Source: CAD feature listing. Evaluate the final solid. Frame: model axes, mm. Face numbers are marked on the shaded views. A direction names the side the tool comes from. Give positions to 0.01 mm unless a question says otherwise; leave off trailing zeros. Loops run counter-clockwise (first coordinate to the right, second up) from the corner with the lowest first, then second, coordinate; pieces in that order, holes last.
from build123d import *

# Parameters (mm, degrees)
IZIM1_R                     = 25
IZIM1_R_2                   = 7.5
Y_KSEKLIK_EKSTR_ZYON1_DEPTH = 80.5
IZIM2_R                     = 16
KES_EKSTR_ZYON1_DEPTH       = 9


with BuildPart() as part:
    # Çizim1 → Yükseklik-Ekstrüzyon1 (new, symmetric)
    with BuildSketch(Plane(origin=(0, 0, 0), x_dir=(0, 0, -1), z_dir=(1, 0, 0))):
        Circle(IZIM1_R)
        Circle(IZIM1_R_2, mode=Mode.SUBTRACT)
    extrude(amount=Y_KSEKLIK_EKSTR_ZYON1_DEPTH, both=True)

    # Çizim2 → Kes-Ekstrüzyon1 (cut)
    with BuildSketch(Plane(origin=(80.5, 0, 0), x_dir=(0, 0, -1), z_dir=(1, 0, 0))):
        Circle(IZIM2_R)
    kes_ekstr_zyon1 = extrude(amount=-KES_EKSTR_ZYON1_DEPTH, mode=Mode.SUBTRACT)

    # Aynalama1: Kes-Ekstrüzyon1 across plane
    add(kes_ekstr_zyon1.mirror(Plane(origin=(0, 0, 0), x_dir=(0, 0, 1), z_dir=(1, 0, 0))), mode=Mode.SUBTRACT)


solid = part.part
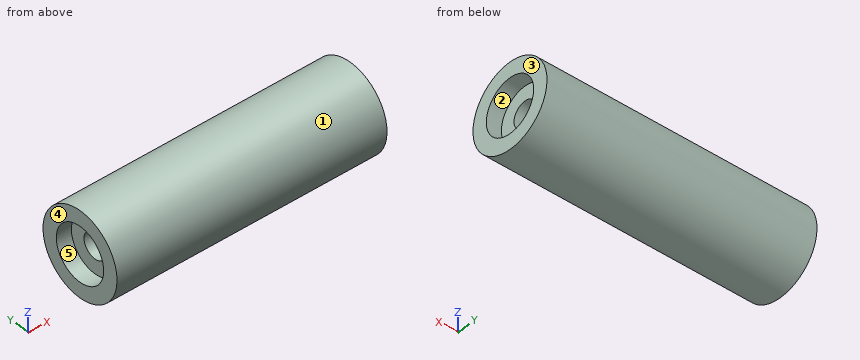
1) Pull-direction query (Z, two-part tool) for the marked faces 1, 2 and 3; classes: released by +Z, released by -Z, zero draft, split by the parting line, or undercut.
Checks:
face 1: split by the parting line
face 2: undercut
face 3: zero draft
2) Reachability of the marked faces 4 and 5 from +Z, -Z, +X, -X, +Y, -Y: full face, straight path, thin tool, end or side. Return the list, or none.
Checks:
face 4: +Z, -Z, -X, +Y, -Y
face 5: -X
3) Ray query, probe 1 along Y at (x, z) = (11.5, 0); probe 2 along Y at (x, z) = (-73, 0); probe 3 along X at (y, z) = (0.5, -13.5). Return the intervals inside material, ascending.
Checks:
probe 1: y = -25 to -7.5, 7.5 to 25
probe 2: y = -25 to -16, 16 to 25
probe 3: x = -71.5 to 71.5
4) Cut plane A-A (z = 0). Return loops of the section in (x, y).
Checks:
outline: (-80.5, -25) - (80.5, -25) - (80.5, -16) - (71.5, -16) - (71.5, -7.5) - (-71.5, -7.5) - (-71.5, -16) - (-80.5, -16) - close; (-80.5, 16) - (-71.5, 16) - (-71.5, 7.5) - (71.5, 7.5) - (71.5, 16) - (80.5, 16) - (80.5, 25) - (-80.5, 25) - close
5) Cut plane D-D (y = -14). Return loops of the section in (x, z).
Checks:
outline: (-80.5, -20.71) - (80.5, -20.71) - (80.5, -7.75) - (71.5, -7.75) - (71.5, 7.75) - (80.5, 7.75) - (80.5, 20.71) - (-80.5, 20.71) - (-80.5, 7.75) - (-71.5, 7.75) - (-71.5, -7.75) - (-80.5, -7.75) - close
6) Contact query for flat-ended pins moving along their axis: P1, Ø2, axis at x = -11.5, z = -11, coming from the +Y side; P2, Ø3, axis at x = 23.5, y = -4.5, coming from the -Z side; P3, Ø19.5, axis at y = 0, z = 0, coming from the -X side. Output: stop coordinate, or through.
Checks:
P1: stops at y = 22.91
P2: stops at z = -24.82
P3: stops at x = -71.5
7) Cut plane C-C (x = 61). Return loops of the section in (y, z), and give its area (3 significant figures).
Checks:
outline: circle Ø50 at (0, 0); hole circle Ø15 at (0, 0)
area: 1,790 mm2
